from build123d import *

# Parameters (mm, degrees)
F0_W     = 127
F0_H     = 50.8
F0_R     = 25.4
F1_DEPTH = 3.175


with BuildPart() as f1:
    # F0 (on Front) → F1 (new body)
    with BuildSketch(Plane.XZ):
        with BuildLine():
            ThreePointArc((0, 6.35), (1.859872, 1.859872), (6.35, 0))
            Line((6.35, 0), (381, 0))
            ThreePointArc((381, 0), (385.490128, 1.859872), (387.35, 6.35))
            Line((387.35, 6.35), (387.35, 374.65))
            ThreePointArc((387.35, 374.65), (385.490128, 379.140128), (381, 381))
            Line((381, 381), (6.35, 381))
            ThreePointArc((6.35, 381), (1.859872, 379.140128), (0, 374.65))
            Line((0, 374.65), (0, 6.35))
        make_face()
        with Locations((203.2, 50.8)):
            Rectangle(F0_W, F0_H, mode=Mode.SUBTRACT)
        with Locations((336.55, 190.5)):
            Circle(F0_R, mode=Mode.SUBTRACT)
    extrude(amount=F1_DEPTH)


solid = f1.part
The model under review builds one solid part; all positions refer to its coordinate system, in mm. Round coordinates to 2 decimals unless told otherwise and drop trailing zeros. Loops run counter-clockwise (first coordinate to the right, second up) from the corner with the lowest first, then second, coordinate; pieces in that order, holes last. Notation, with made-up numbers: M -26.75,85 L -21.75,85 A15 ccw -21.75,94 Z; hole C 70,37.25 d5. An arc over 180 degrees is marked long. Answer as CSV lines item,"result". Start each with the question number.
Item 1: Consider section C-C (y = -0.95). Write out the cut boundary in (x, z), then the cut area to 3 significant figures.
Item 2: Consider section A-A (x = 336.55). Write out the cut boundary in (y, z) (3 decimals), then the cut area to 3 significant figures.
Item 3: Wall thickness on line 1 (Z direction, x = 336.55, y = -2.1); line 2 (X direction, y = -2.9, z = 59.5); line 3 (Z direction, x = 242.5, y = -0.75): over which ranges is each line inside the solid? List them lowest first. Write a range as [from, to].
Item 4: Consider section B-B (z = 190.5). Write out the cut boundary in (x, y) (3 decimals).
Item 5: Mouldability with a two-part tool opening along Z and no side actions: class faces 1 (the face through (191, 0, 193)), 2 (the face through (316.393, -1.565, 175.044)) as released by +Z, released by -Z, zero draft, split by the parting line, or undercut.
Answer:
1,outline,"M 0,6.35 A6.35 ccw 6.35,0 L 381,0 A6.35 ccw 387.35,6.35 L 387.35,374.65 A6.35 ccw 381,381 L 6.35,381 A6.35 ccw 0,374.65 Z; hole M 139.7,25.4 L 266.7,25.4 L 266.7,76.2 L 139.7,76.2 Z; hole C 336.55,190.5 d50.8"
1,area,"139,000 mm^2"
2,outline,"M -3.175,0 L 0,0 L 0,165.1 L -3.175,165.1 Z; M -3.175,215.9 L 0,215.9 L 0,381 L -3.175,381 Z"
2,area,"1,050 mm^2"
3,line 1,"z = [0, 165.1], [215.9, 381]"
3,line 2,"x = [0, 139.7], [266.7, 387.35]"
3,line 3,"z = [0, 25.4], [76.2, 381]"
4,outline,"M 0,-3.175 L 311.15,-3.175 L 311.15,0 L 0,0 Z; M 361.95,-3.175 L 387.35,-3.175 L 387.35,0 L 361.95,0 Z"
5,face 1,"zero draft"
5,face 2,"undercut"
